Verification items for the finished model (mm, model axes). Face numbers are marked on the shaded views. A direction names the side the tool comes from. Round coordinates to 2 decimals unless told otherwise and drop trailing zeros. Write each loop counter-clockwise with the first axis right and the second up, starting at its lowest first coordinate (ties: lowest second). Pieces come first, ordered by that corner, then holes. Notation, with made-up numbers: M 67.25,3 L 123.25,3 A21 cw 123.25,25 Z; hole C -17.75,43.5 d7. An arc over 180 degrees is marked long. Answer in a Markdown table with one row per item. Add a question column.
1. Draft check along Z on the marked faces 1, 2, 3 and 4. Enter one of: pulls with the +Z half, pulls with the -Z half, needs draft (parallel to the pull), parting line crosses it, or undercut.
2. Sectioned sample at C-C on z = 4.25. Record the cut outline in (x, y), plus the area to 3 significant figures.
3. Sectioned sample at D-D on z = 16.5. Record the cut outline in (x, y), plus the area to 3 significant figures.
4. Set-up check for the marked faces 5, 6 and 7: record each of +Z, -Z, +X, -X, +Y, -Y from which the full face is reachable in a straight line by a thin tool's end or side.
5. Go/stop test with flat-tipped pins: pin 1 Ø2 at (x, z) = (-2.5, 2.5) entering from -Y; pin 2 Ø3 at (x, z) = (2.5, 13.5) entering from -Y; pin 3 Ø3 at (y, z) = (-4.5, 10.5) entering from -X; pin 4 Ø4 at (y, z) = (-0.5, 9.5) entering from -X. Record where each tip stops, or that it passes through.
6. Material ranges on probe 1 along Y at (x, z) = (0, 2.05); probe 2 along Z at (x, y) = (5, 2.75); probe 3 along Z at (x, y) = (-3.25, -2.5), recorded low to high.
7. Sectioned sample at A-A on y = 0. Record the cut outline in (x, z) (3 decimals), plus the area to 3 significant figures.
```python
from build123d import *


with BuildPart() as f1:
    # F0 (on Front) → F1 (revolve)
    with BuildSketch(Plane.XZ):
        Polygon((0, 7), (0, 5), (0.85, 5), (0.85, 0), (4.85, 0), (4.85, 5), (6.85, 5), (6.85, 7), (3.425, 7), align=None)
        Polygon((0, 22), (0, 7), (3.425, 7), (1.750177, 17.936636), (2.5, 20.5), (2.5, 22), align=None)
    revolve(axis=Axis((0, 0, 15.337315), (0, 0, 1)))


solid = f1.part
```
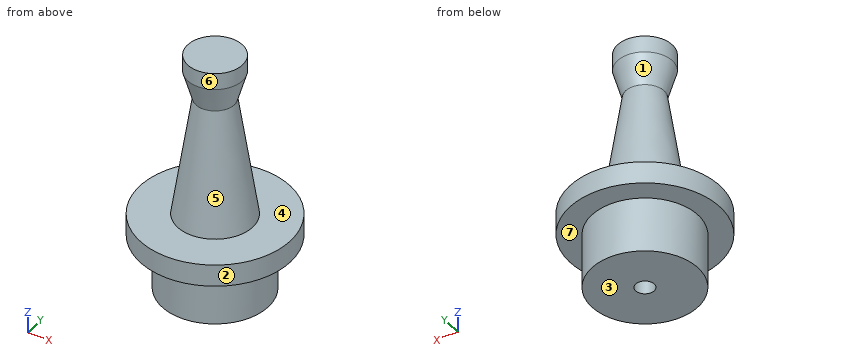
Geometry check:
| question | item | result |
|---|---|---|
| 1 | face 1 | undercut |
| 1 | face 2 | needs draft |
| 1 | face 3 | pulls with the -Z half |
| 1 | face 4 | pulls with the +Z half |
| 2 | outline | C 0,0 d9.7; hole C 0,0 d1.7 |
| 2 | area | 71.6 mm2 |
| 3 | outline | C 0,0 d3.94 |
| 3 | area | 12.2 mm2 |
| 4 | face 5 | none |
| 4 | face 6 | +Z |
| 4 | face 7 | -Z |
| 5 | pin 1 | stops at y = -4.61 |
| 5 | pin 2 | stops at y = -2.26 |
| 5 | pin 3 | passes through |
| 5 | pin 4 | stops at x = -3.34 |
| 6 | probe 1 | y = -4.85 to -0.85, 0.85 to 4.85 |
| 6 | probe 2 | z = 5 to 7 |
| 6 | probe 3 | z = 0 to 7 |
| 7 | outline | M -6.85,5 L -4.85,5 L -4.85,0 L -0.85,0 L -0.85,5 L 0.85,5 L 0.85,0 L 4.85,0 L 4.85,5 L 6.85,5 L 6.85,7 L 3.425,7 L 1.75,17.937 L 2.5,20.5 L 2.5,22 L -2.5,22 L -2.5,20.5 L -1.75,17.937 L -3.425,7 L -6.85,7 Z |
| 7 | area | 142 mm2 |
